For this review, use the dimensioned drawing (mm, ordinates from the lowest corner) and the shaded views. Round coordinates to 2 decimals unless told otherwise and drop trailing zeros. Write each loop counter-clockwise with the first axis right and the second up, starting at its lowest first coordinate (ties: lowest second). Pieces come first, ordered by that corner, then holes. Notation, with made-up numbers: (21, 68) - (75, 68) arc R20 ccw to (75, 87) - close; hole circle Ø2 at (85.5, 38). An arc over 180 degrees is marked (long way). Return JSON: item names as keys, results as strings.
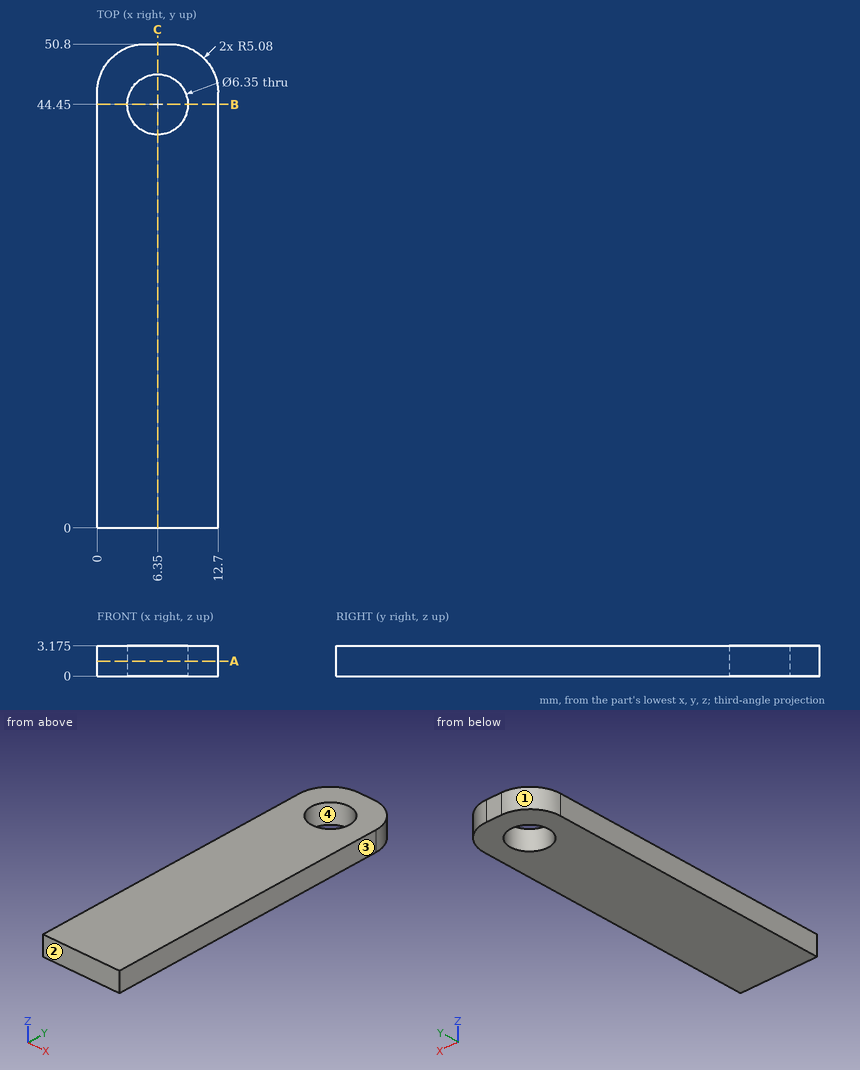
(1) Add section C-C (x = 6.35). Write out the cut boundary in (y, z) (3 decimals).
Filled in:
{"outline": "(0, 0) - (41.275, 0) - (41.275, 3.175) - (0, 3.175) - close; (47.625, 0) - (50.8, 0) - (50.8, 3.175) - (47.625, 3.175) - close"}
(2) Add section A-A (z = 1.55). Write out the cut boundary in (x, y) (3 decimals), plus the area to 3 significant figures.
Filled in:
{"outline": "(0, 0) - (12.7, 0) - (12.7, 45.72) arc R5.08 ccw to (7.62, 50.8) - (5.08, 50.8) arc R5.08 ccw to (0, 45.72) - close; hole circle Ø6.35 at (6.35, 44.45)", "area": "602 mm2"}
(3) Wall thickness on line 1 (Y direction, x = 6.35, z = 2.55) (3 decimals); line 2 (Y direction, x = 3.75, z = 1.8); line 3 (X direction, y = 49, z = 2.2): over which ranges is each line inside the solid? List them lowest first.
Filled in:
{"line 1": "y = 0 to 41.275, 47.625 to 50.8", "line 2": "y = 0 to 42.63, 46.27 to 50.62", "line 3": "x = 1.2 to 11.5"}
(4) Mouldability with a two-part tool opening along X and no side actions: class the marked faces 1, 2, 3 and 4 as released by +X, released by -X, zero draft, split by the parting line, or undercut.
Filled in:
{"face 1": "released by -X", "face 2": "zero draft", "face 3": "released by +X", "face 4": "undercut"}
(5) Add section B-B (y = 44.45). Write out the cut boundary in (x, z) (3 decimals).
Filled in:
{"outline": "(0, 0) - (3.175, 0) - (3.175, 3.175) - (0, 3.175) - close; (9.525, 0) - (12.7, 0) - (12.7, 3.175) - (9.525, 3.175) - close"}
